For this review, take the finished solid that the model builds, in its own axes (mm). Face numbers are marked on the shaded views. A direction names the side the tool comes from. Coordinates: 2 decimals unless noted, no trailing zeros. Order: outer loops, then holes, each group sorted by start corner. A loop starts at its lowest first (then second) coordinate and runs counter-clockwise, first axis right, second up. Notation, with made-up numbers: (6, 84.25) -> (38, 84.25) arc R28 cw to (38, 116.25) -> close; hole circle Ø1 at (87, -19.75). An arc over 180 degrees is marked (long way). Answer as a JSON object with one key per item and string values. Group by question number.
1) Add section C-C, the plane y = 0. Write out the cut boundary in (x, z).
2) Wall thickness on L1, parallel to Y at x = -24.1, z = 2.2; L2, parallel to X at y = -10.5, z = 1.5; L3, parallel to Z at x = 22, y = -20: over which ranges is each line inside the solid? List them lowest first.
3) For pin 1 (0.9 mm diameter, centred on x = 31, z = -6, fed in from +Y); pin 2 (3 mm diameter, centred on y = 4, z = -3, fed in from -X); pin 3 (1.5 mm diameter, centred on x = 30.5, z = -16.5, fed in from -Y); pin 4 (8 mm diameter, centred on x = 35, y = -23, fed in from +Z), all flat-tipped, find the tip position at first contact; note any pin that passes through.
4) Add section B-B, the plane x = -24.1. Write out the cut boundary in (y, z).
5) Machinability: for the marked faces 1, 2 and 3, which of the approach directions +Z, -Z, +X, -X, +Y, -Y give a long, thin tool a straight path to every point of the face, cutting with its end or side? Answer none if there is none.
6) Add section D-D, the plane x = 46.5. Write out the cut boundary in (y, z).
7) Add section A-A, the plane y = 12. Write out the cut boundary in (x, z), then the cut area to 3 significant figures.
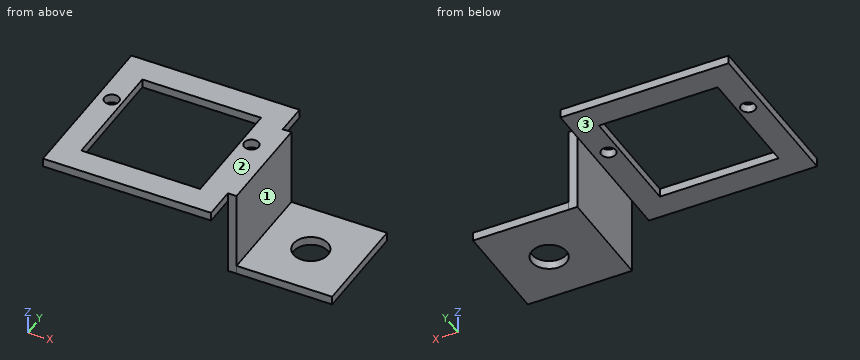
from build123d import *

# Parameters (mm, degrees)
F0_W     = 58
F0_H     = 58
F0_R     = 2.5
F0_W_2   = 41
F0_H_2   = 40
F1_DEPTH = 3
F2_W     = 36
F2_H     = 27
F2_H_2   = 3
F3_DEPTH = 3
F4_W     = 33
F4_H     = 35.972737
F4_R     = 6
F5_DEPTH = 3


with BuildPart() as f1:
    # F0 (on Top) → F1 (new body)
    with BuildSketch(Plane.XY):
        Rectangle(F0_W, F0_H)
        with Locations((-24.1, 6.807183)):
            Circle(F0_R, mode=Mode.SUBTRACT)
        Rectangle(F0_W_2, F0_H_2, mode=Mode.SUBTRACT)
        with Locations((24.1, 6.807183)):
            Circle(F0_R, mode=Mode.SUBTRACT)
    extrude(amount=F1_DEPTH)

    # F2 (on face) → F3 (join)
    with BuildSketch(Plane.YZ.offset(29)):
        with Locations((0.023433, -13.5)):
            Rectangle(F2_W, F2_H)
        with Locations((0.023433, 1.5)):
            Rectangle(F2_W, F2_H_2)
    extrude(amount=F3_DEPTH)

    # F4 (on face) → F5 (join)
    with BuildSketch(Plane(origin=(0, 0, -27), x_dir=(1, 0, 0), z_dir=(0, 0, -1))):
        with Locations((48.5, -0.009802)):
            Rectangle(F4_W, F4_H)
        with Locations((48.182182, 0)):
            Circle(F4_R, mode=Mode.SUBTRACT)
    extrude(amount=-F5_DEPTH)


solid = f1.part
Output values:
{
 "1": {"outline": "(-29, 0) -> (-20.5, 0) -> (-20.5, 3) -> (-29, 3) -> close; (20.5, 0) -> (29, 0) -> (29, -27) -> (42.18, -27) -> (42.18, -24) -> (32, -24) -> (32, 3) -> (20.5, 3) -> close; (54.18, -27) -> (65, -27) -> (65, -24) -> (54.18, -24) -> close"},
 "2": {"L1": "y = -29 to 4.31, 9.31 to 29", "L2": "x = -29 to -20.5, 20.5 to 32", "L3": "z = 0 to 3"},
 "3": {"pin 1": "stops at y = 18.02", "pin 2": "stops at x = 29", "pin 3": "stops at y = -17.98", "pin 4": "passes through"},
 "4": {"outline": "(-29, 0) -> (4.31, 0) -> (4.31, 3) -> (-29, 3) -> close; (9.31, 0) -> (29, 0) -> (29, 3) -> (9.31, 3) -> close"},
 "5": {"face 1": "+Z, +X, +Y, -Y", "face 2": "+Z, +X, -X, +Y, -Y", "face 3": "-Z, -X, +Y, -Y"},
 "6": {"outline": "(-17.98, -27) -> (-5.76, -27) -> (-5.76, -24) -> (-17.98, -24) -> close; (5.76, -27) -> (18, -27) -> (18, -24) -> (5.76, -24) -> close"},
 "7": {"outline": "(-29, 0) -> (-20.5, 0) -> (-20.5, 3) -> (-29, 3) -> close; (20.5, 0) -> (29, 0) -> (29, -27) -> (65, -27) -> (65, -24) -> (32, -24) -> (32, 3) -> (20.5, 3) -> close", "area": "240 mm²"}
}
